Geometry: final body of the model. Coordinates: model frame, mm. A direction names the side the tool comes from. Give positions to 0.01 mm unless a question says otherwise; leave off trailing zeros. Write each loop counter-clockwise with the first axis right and the second up, starting at its lowest first coordinate (ties: lowest second). Pieces come first, ordered by that corner, then holes. Notation, with made-up numbers: (29.5, 87.25) -> (81.5, 87.25) arc R12 cw to (81.5, 101.25) -> close; hole circle Ø5 at (-15, 63.25). An arc over 180 degrees is marked (long way). Answer in a Markdown table with one row per item. Add a question column.
Item 1: Section query B-B on z = 14.5. Output: boundary loops of the cut face in (x, y).
Item 2: Material intervals for probe 1 along Y at (x, z) = (-0.25, 27); probe 2 along Z at (x, y) = (-3, 49); probe 3 along X at (y, z) = (54, 25.5), sorted ascending. Write a range as from..to.
Item 3: Section query C-C on y = 21. Output: boundary loops of the cut face in (x, z).
Item 4: First-contact query: P1, Ø2, axis at x = 3, z = 4.5, coming from the -Y side; P2, Ø1, axis at x = -3, y = 88, coming from the +Z side; P3, Ø3, axis at x = -1.5, z = 25, coming from the -Y side; P4, Ø6, axis at x = -3, y = 104.5, coming from the -Z side. Flat tips, straight axial feed; report the tip coordinate or a pass-through.
Item 5: Access query for faces 1 (the cylindrical face through (-4.43, 50.6, 12.33)), 2 (the flat face through (5, 86, 13)), 3 (the cylindrical face through (4.43, 50.6, 12.68)). Directions: +Z, -Z, +X, -X, +Y, -Y. A direction counts if a zero-diameter tool reaches every point of the face in a straight line with its end or side. Return the directions, or none.
```python
from build123d import *

# Parameters (mm, degrees)
SKETCH1_R           = 5
BOSS_EXTRUDE1_DEPTH = 50
BOSS_EXTRUDE2_DEPTH = 70
FILLET1_R           = 5
FILLET2_R           = 2
FILLET3_R           = 2


# Some blends are built 0.0001 mm under size
with BuildPart() as part:
    # Sketch1 → Boss-Extrude1 (new body)
    with BuildSketch(Plane(origin=(0, 0, 0), x_dir=(1, 0, 0), z_dir=(0, 1, 0))):
        with Locations(Location((0, 0, 0), (0, 0, 270))):
            Circle(SKETCH1_R)
    extrude(amount=BOSS_EXTRUDE1_DEPTH)

    # Sketch2 → Boss-Extrude2 (add)
    with BuildSketch(Plane(origin=(0, 50, 0), x_dir=(1, 0, 0), z_dir=(0, 1, 0))):
        with BuildLine():
            Line((-5, 0), (-5, -30))
            Line((-5, -30), (5, -30))
            Line((5, -30), (5, 0))
            ThreePointArc((5, 0), (0, 5), (-5, 0))
        make_face()
    extrude(amount=BOSS_EXTRUDE2_DEPTH)

    # Fillet1
    fillet1_edges = [part.edges().sort_by_distance(p)[0] for p in [
        (-5, 85, 30),
        (5, 85, 30),
    ]]
    fillet(fillet1_edges, radius=FILLET1_R - 0.0001)  # a hair under: the kernel refuses the full size

    # Fillet2
    # the kernel refuses this fillet: 2 mm, written as the material it takes off along each edge
    with BuildSketch(Plane(origin=(5, 50, 25.0001), x_dir=(-1, 0, 0), z_dir=(0, 0, -1))) as fillet2_piece_1_section:
        with BuildLine():
            CenterArc((FILLET2_R, FILLET2_R), FILLET2_R, 180, 90)
            Line((0, FILLET2_R), (0, 0))
            Line((0, 0), (FILLET2_R, 0))
        make_face()
    fillet2_piece_1 = extrude(amount=30.0001, mode=Mode.PRIVATE)
    fillet2_piece_1 = fillet2_piece_1 - Plane(origin=(0, 50.338854102, 0), x_dir=(0, 0, 1), z_dir=(0, -1, 0)) * Cylinder(5, 69, mode=Mode.PRIVATE)
    add(fillet2_piece_1, mode=Mode.SUBTRACT)
    with BuildSketch(Plane(origin=(0.0001, 50, 25.0001), x_dir=(1, 0, 0), z_dir=(0, 0, -1))) as fillet2_piece_2:
        with BuildLine():
            CenterArc((4.9999 - FILLET2_R, -FILLET2_R), FILLET2_R, 0, 90)
            Line((4.9999, -FILLET2_R), (4.9999, 0))
            Line((4.9999, 0), (4.9999 - FILLET2_R, 0))
        make_face()
    revolve(axis=Axis((0.0001, 50, 25.0001), (0, -1, 0)), revolution_arc=90, mode=Mode.SUBTRACT)
    with BuildSketch(Plane(origin=(-0.0001, 50, 25.0001), x_dir=(0, 0, 1), z_dir=(1, 0, 0))) as fillet2_piece_3:
        with BuildLine():
            CenterArc((4.9999 - FILLET2_R, -FILLET2_R), FILLET2_R, 0, 90)
            Line((4.9999, -FILLET2_R), (4.9999, 0))
            Line((4.9999, 0), (4.9999 - FILLET2_R, 0))
        make_face()
    revolve(axis=Axis((-0.0001, 50, 25.0001), (0, -1, 0)), revolution_arc=90, mode=Mode.SUBTRACT)
    with BuildSketch(Plane(origin=(-5, 50, -5), x_dir=(1, 0, 0), z_dir=(0, 0, 1))) as fillet2_piece_4_section:
        with BuildLine():
            CenterArc((FILLET2_R, FILLET2_R), FILLET2_R, 180, 90)
            Line((0, FILLET2_R), (0, 0))
            Line((0, 0), (FILLET2_R, 0))
        make_face()
    fillet2_piece_4 = extrude(amount=30.0001, mode=Mode.PRIVATE)
    fillet2_piece_4 = fillet2_piece_4 - Plane(origin=(0, 50.465433579, 0), x_dir=(0, 0, 1), z_dir=(0, -1, 0)) * Cylinder(5, 69, mode=Mode.PRIVATE)
    add(fillet2_piece_4, mode=Mode.SUBTRACT)
    with BuildSketch(Plane(origin=(-0.0001, 50, 30), x_dir=(0, 0, -1), z_dir=(1, 0, 0))) as fillet2_piece_5:
        with BuildLine():
            CenterArc((FILLET2_R, FILLET2_R), FILLET2_R, 180, 90)
            Line((0, FILLET2_R), (0, 0))
            Line((0, 0), (FILLET2_R, 0))
        make_face()
    extrude(amount=0.0002, mode=Mode.SUBTRACT)

    # Fillet3
    fillet3_edges = [part.edges().sort_by_distance(p)[0] for p in [
        (0, 0, -5),
    ]]
    fillet(fillet3_edges, radius=FILLET3_R)


solid = part.part
```
Findings below:
| question | item | result |
|---|---|---|
| 1 | outline | (-5, 52) arc R2 ccw to (-3, 50) -> (3, 50) arc R2 ccw to (5, 52) -> (5, 120) -> (-5, 120) -> close |
| 2 | probe 1 | y = 50..120 |
| 2 | probe 2 | z = -4..4 |
| 2 | probe 3 | x = -4.97..4.97 |
| 3 | outline | circle Ø10 at (0, 0) |
| 4 | P1 | stops at y = 0.58 |
| 4 | P2 | stops at z = 29.33 |
| 4 | P3 | stops at y = 50 |
| 4 | P4 | stops at z = -5 |
| 5 | face 1 | +Z, -X, -Y |
| 5 | face 2 | +Z, -Z, +X, +Y, -Y |
| 5 | face 3 | +Z, +X, -Y |
